Verification items for the finished model (mm, model axes). A direction names the side the tool comes from. Coordinates: 2 decimals unless noted, no trailing zeros. Order: outer loops, then holes, each group sorted by start corner. A loop starts at its lowest first (then second) coordinate and runs counter-clockwise, first axis right, second up. Notation, with made-up numbers: (-0.75, 6) -> (25.25, 6) arc R28 ccw to (25.25, 25) -> close; hole circle Ø4 at (-22, 2.25). An arc over 180 degrees is marked (long way). Write item = value, one per line. Start each with the question number.
1. Cross-section at B-B on y = 0.75. Record the cut outline in (x, z) (3 decimals).
2. Go/stop test with flat-tipped pins: P1, Ø4.5, axis at x = -23.5, y = 2.5, coming from the -Z side; P2, Ø0.9, axis at y = -0.5, z = 0.5, coming from the -X side; P3, Ø0.9, axis at y = -3.5, z = 2, coming from the -X side. Record where each tip stops, or that it passes through.
3. Thickness scan on line 1 along X through (y, z) = (-5.25, -4.25); line 2 along X through (y, z) = (0, -3.25); line 3 along Y through (x, z) = (17.5, 1.5) (3 decimals). Record the ranges inside material, lowest first. Write a range as from..to.
4. Cross-section at D-D on x = 1. Record the cut outline in (y, z) (3 decimals).
5. Set-up check for faces 1 (the flat face through (0, 0, 0)), 2 (the flat face through (-25.6, 6, 1)), 3 (the flat face through (21.6, 0, 2)): record each of +Z, -Z, +X, -X, +Y, -Y from which the full face is reachable in a straight line by a thin tool's end or side.
6. Cross-section at A-A on x = 17.5. Record the cut outline in (y, z) (3 decimals), plus the area to 3 significant figures.
7. Release check for a two-part mould opening along Y. For faces 4 (the flat face through (23, 0, -1.5)), 5 (the flat face through (0, 7.075, 0)), 6 (the flat face through (23.6, 0.1, 0.6)), 7 (the flat face through (-5.4, -4, 2)) record: +Y half, -Y half, draft (parallel to the pull), parting line (faces both ways), or undercut.
8. Cross-section at C-C on z = -5. Record the cut outline in (x, y) (3 decimals), plus the area to 3 significant figures.
from build123d import *

# Parameters (mm, degrees)
F1_DEPTH = 3.15
F0_W     = 47.2
F0_H     = 10.15
F3_DEPTH = 1.5
F4_DEPTH = 2
F2_W     = 4
F2_H     = 2
F5_DEPTH = 1.75
F7_DEPTH = 14.15


with BuildPart() as f1:
    # F0 (on Top) → F1 (new body)
    with BuildSketch(Plane.XY):
        Polygon((23.6, 5.075), (23.6, -5.075), (-23.6, -5.075), (-25.6, -5.075), (-25.6, -7.075), (25.6, -7.075), (25.6, 7.075), (-25.6, 7.075), (-25.6, 5.075), (-23.6, 5.075), align=None)
    extrude(amount=F1_DEPTH)

    # F0 (on Top) → F3 (join)
    with BuildSketch(Plane.XY):
        Rectangle(F0_W, F0_H)
        Polygon((23.6, 5.075), (23.6, -5.075), (-23.6, -5.075), (-25.6, -5.075), (-25.6, -7.075), (25.6, -7.075), (25.6, 7.075), (-25.6, 7.075), (-25.6, 5.075), (-23.6, 5.075), align=None)
    extrude(amount=-F3_DEPTH)

    # F2 (on face) → F4 (join)
    with BuildSketch(Plane.XY.offset(3.15)):
        Polygon((23.6, -5.075), (23.6, -3.075), (21.6, -3.075), (-1.4, -3.075), (-1.4, -5.075), align=None)
        Polygon((23.6, 5.075), (-1.4, 5.075), (-1.4, 3.075), (21.6, 3.075), (21.6, -3.075), (23.6, -3.075), align=None)
    extrude(amount=-F4_DEPTH)

    # F2 (on face) → F5 (join)
    with BuildSketch(Plane.XY.offset(3.15)):
        with Locations((-3.4, -4.075)):
            Rectangle(F2_W, F2_H)
        with Locations((-3.4, 4.075)):
            Rectangle(F2_W, F2_H)
    extrude(amount=-F5_DEPTH)

    # F6 (on face) → F7 (join)
    with BuildSketch(Plane(origin=(0, 7.075, 0), x_dir=(-1, 0, 0), z_dir=(0, 1, 0))):
        with BuildLine():
            Line((12.0083426132, -1.5), (11.812996063, -1.5))
            ThreePointArc((11.812996063, -1.5), (14.2379267863, -9.0095722129), (20.625, -4.375))
            ThreePointArc((20.625, -4.375), (20.3845722129, -2.8629267863), (19.687003937, -1.5))
            Line((19.687003937, -1.5), (19.4916573868, -1.5))
            Line((19.4916573868, -1.5), (18.25, -1.5))
            Line((18.25, -1.5), (15.75, -1.5))
            Line((15.75, -1.5), (12.0083426132, -1.5))
        make_face()
        with BuildLine():
            ThreePointArc((18.625, -4.375), (13.7170680041, -6.4079319959), (15.75, -1.5))
            ThreePointArc((15.75, -1.5), (17.7829319959, -2.3420680041), (18.625, -4.375))
        make_face(mode=Mode.SUBTRACT)
        with BuildLine():
            ThreePointArc((13.5994186832, 0), (12.615167699, -0.6415764445), (11.812996063, -1.5))
            Line((11.812996063, -1.5), (12.0083426132, -1.5))
            Line((12.0083426132, -1.5), (15.75, -1.5))
            Line((15.75, -1.5), (18.25, -1.5))
            Line((18.25, -1.5), (19.4916573868, -1.5))
            Line((19.4916573868, -1.5), (19.687003937, -1.5))
            ThreePointArc((19.687003937, -1.5), (18.884832301, -0.6415764445), (17.9005813168, 0))
            Line((17.9005813168, 0), (17.8115528128, 0))
            Line((17.8115528128, 0), (13.6884471872, 0))
            Line((13.6884471872, 0), (13.5994186832, 0))
        make_face()
        with BuildLine():
            Line((-19.4916573868, -1.5), (-18.25, -1.5))
            Line((-18.25, -1.5), (-15.75, -1.5))
            Line((-15.75, -1.5), (-12.0083426132, -1.5))
            Line((-12.0083426132, -1.5), (-11.812996063, -1.5))
            ThreePointArc((-11.812996063, -1.5), (-12.615167699, -0.6415764445), (-13.5994186832, 0))
            Line((-13.5994186832, 0), (-13.6884471872, 0))
            Line((-13.6884471872, 0), (-17.8115528128, 0))
            Line((-17.8115528128, 0), (-17.9005813168, 0))
            ThreePointArc((-17.9005813168, 0), (-18.884832301, -0.6415764445), (-19.687003937, -1.5))
            Line((-19.687003937, -1.5), (-19.4916573868, -1.5))
        make_face()
        with BuildLine():
            Line((-15.75, -1.5), (-18.25, -1.5))
            Line((-18.25, -1.5), (-19.4916573868, -1.5))
            Line((-19.4916573868, -1.5), (-19.687003937, -1.5))
            ThreePointArc((-19.687003937, -1.5), (-17.2620732137, -9.0095722129), (-10.875, -4.375))
            ThreePointArc((-10.875, -4.375), (-11.1154277871, -2.8629267863), (-11.812996063, -1.5))
            Line((-11.812996063, -1.5), (-12.0083426132, -1.5))
            Line((-12.0083426132, -1.5), (-15.75, -1.5))
        make_face()
        with BuildLine():
            ThreePointArc((-12.875, -4.375), (-17.7829319959, -6.4079319959), (-15.75, -1.5))
            ThreePointArc((-15.75, -1.5), (-13.7170680041, -2.3420680041), (-12.875, -4.375))
        make_face(mode=Mode.SUBTRACT)
    extrude(amount=-F7_DEPTH)


solid = f1.part
Worked out:
q1.outline = (-23.6, -1.5) -> (-19.687, -1.5) arc R4.875 ccw (long way) to (-11.813, -1.5) -> (11.813, -1.5) arc R4.875 ccw (long way) to (19.687, -1.5) -> (25.6, -1.5) -> (25.6, 3.15) -> (21.6, 3.15) -> (21.6, 1.15) -> (23.6, 1.15) -> (23.6, 0) -> (-23.6, 0) -> close; hole circle Ø5.75 at (-15.75, -4.375); hole circle Ø5.75 at (15.75, -4.375)
q2.P1 = -1.5
q2.P2 = 23.6
q2.P3 = -5.4
q3.line_1 = -20.62..-18.62, -12.88..-10.88, 10.88..12.88, 18.62..20.62
q3.line_2 = -20.49..-18.4, -13.1..-11.01, 11.01..13.1, 18.4..20.49
q3.line_3 = -7.075..-3.075, 3.075..7.075
q4.outline = (-7.075, -1.5) -> (7.075, -1.5) -> (7.075, 3.15) -> (3.075, 3.15) -> (3.075, 1.15) -> (5.075, 1.15) -> (5.075, 0) -> (-5.075, 0) -> (-5.075, 1.15) -> (-3.075, 1.15) -> (-3.075, 3.15) -> (-7.075, 3.15) -> close
q5.face_1 = -X
q5.face_2 = +Z, -Z, -X, +Y, -Y
q5.face_3 = +Z, -X
q6.outline = (-7.075, -8.925) -> (7.075, -8.925) -> (7.075, -6.656) -> (-7.075, -6.656) -> close; (-7.075, -2.094) -> (7.075, -2.094) -> (7.075, 3.15) -> (3.075, 3.15) -> (3.075, 1.15) -> (5.075, 1.15) -> (5.075, 0) -> (-5.075, 0) -> (-5.075, 1.15) -> (-3.075, 1.15) -> (-3.075, 3.15) -> (-7.075, 3.15) -> close
q6.area = 82.3 mm²
q7.face_4 = draft
q7.face_5 = +Y half
q7.face_6 = undercut
q7.face_7 = undercut
q8.outline = (-20.585, -7.075) -> (-18.556, -7.075) -> (-18.556, 7.075) -> (-20.585, 7.075) -> close; (-12.944, -7.075) -> (-10.915, -7.075) -> (-10.915, 7.075) -> (-12.944, 7.075) -> close; (10.915, -7.075) -> (12.944, -7.075) -> (12.944, 7.075) -> (10.915, 7.075) -> close; (18.556, -7.075) -> (20.585, -7.075) -> (20.585, 7.075) -> (18.556, 7.075) -> close
q8.area = 115 mm²
